Autodesk Inventor part; units mm, degrees
ref_plane "YZ Plane" through (0, 0, 0) normal (1, 0, 0) x (0, 1, 0)
ref_plane "XZ Plane" through (0, 0, 0) normal (0, 1, 0) x (-1, 0, 0)
ref_plane "XY Plane" through (0, 0, 0) normal (0, 0, 1) x (1, 0, 0)
sketch "Sketch1" plane through (0, 0, 0) normal (0, 1, 0) x (-1, 0, 0)
  arc A0 (-2.05, -2.3917) -> (-2.05, 2.3917) centre (0, 0) ccw
  line L0 (3.15, 0) -> (-2.05, 0)
  line L1 (-2.05, 0) -> (-2.05, -2.3917)
  line L2 (-2.05, 0) -> (-2.05, 2.3917)
  circle A1 centre (0, 0) radius 8
  dimension "d0" = 6.3
  dimension "d1" = 5.2
  dimension "d2" = 16
extrude "Extrusion1" add sketch "Sketch1" along normal blind 10
sketch "Sketch2" plane through (0, 10, 0) normal (0, 1, 0) x (1, 0, 0)
  arc A0 (2.05, 2.3917) -> (2.05, -2.3917) centre (0, 0) ccw
  line L0 (2.05, 2.3917) -> (2.05, -2.3917)
extrude "Extrusion2" add sketch "Sketch2" against normal blind 1
sketch "Sketch3" plane through (0, 0, 0) normal (0, -1, 0) x (1, 0, 0)
  arc A0 (2.05, 2.3917) -> (2.05, -2.3917) centre (0, 0) ccw
  line L0 (2.05, 2.3917) -> (2.05, -2.3917)
  circle A1 centre (0, 0) radius 7
  dimension "d7" = 14
extrude "Extrusion3" cut sketch "Sketch3" against normal blind 6
sketch "Sketch4" plane through (0, 0, 0) normal (0, -1, 0) x (1, 0, 0)
  circle A0 centre (0, 0) radius 8
  circle A1 centre (0, 0) radius 12
  dimension "d10" = 24
extrude "Extrusion4" add sketch "Sketch4" against normal blind 3
fillet "Fillet1" radius 4 3 edges at (8, 3, 0) (-12, 3, 0) (8, 10, 0)
properties part number "galka enkodera"
Geometry check sheet. Reference: the model listing, model coordinates, mm. A direction names the side the tool comes from. Give positions to 0.01 mm unless a question says otherwise; leave off trailing zeros. Write each loop counter-clockwise with the first axis right and the second up, starting at its lowest first coordinate (ties: lowest second). Pieces come first, ordered by that corner, then holes.
1) Release check for a two-part mould opening along Z. For faces 3 (the face through (0, 10, 0)), 4 (the face through (2.05, 7, 0)) record: released by +Z, released by -Z, zero draft, split by the parting line, or undercut.
Values follow:
face 3: zero draft
face 4: undercut
2) Go/stop test with flat-tipped pins: pin 1 Ø8 at (x, z) = (0, 0) entering from -Y; pin 2 Ø6 at (x, y) = (-0.5, 5) entering from +Z; pin 3 Ø1.5 at (y, z) = (7, 1) entering from -X. Record where each tip stops, or that it passes through.
Values follow:
pin 1: stops at y = 6
pin 2: stops at z = 11.5
pin 3: stops at x = -8.03
3) Thickness scan on line 1 (Z direction, x = 0, y = 6.85); line 2 (Z direction, x = 1.5, y = 5.5); line 3 (X direction, y = 8, z = 0.25). Record the ranges inside material, lowest first.
Values follow:
line 1: z = -7.97 to -3.15, 3.15 to 7.97
line 2: z = -8.16 to -6.84, 6.84 to 8.16
line 3: x = -7.52 to -3.14, 2.05 to 7.52
4) Cross-section at A-A (y = 2). Record the boundary of the cut face in (x, z), plus the area to 3 significant figures.
Values follow:
outline: circle Ø23.01 at (0, 0); hole circle Ø14 at (0, 0)
area: 262 mm2
5) Set-up check for faces 1 (the face through (5.2, 0, -5.2)), 2 (the face through (6.466, 2.958, -2.681)): record each of +Z, -Z, +X, -X, +Y, -Y from which the full face is reachable in a straight line by a thin tool's end or side.
Values follow:
face 1: +Z, -Z, +X, -X, -Y
face 2: -Y
6) Cross-section at B-B (y = 4). Record the boundary of the cut face in (x, z), plus the area to 3 significant figures.
Values follow:
outline: circle Ø18.71 at (0, 0); hole circle Ø14 at (0, 0)
area: 121 mm2
